from build123d import *

# Parameters (mm, degrees)
F0_R     = 10
F1_DEPTH = 30


with BuildPart() as f1:
    # F0 (on Front) → F1 (new body)
    with BuildSketch(Plane.XZ):
        Polygon((21.585897, 21.436766), (1.585897, 21.436766), (1.585897, 1.436766), (-16.747437, 1.436766), (-16.747437, -18.563234), (53.252563, -18.563234), (53.252563, -3.563234), (47.679901, 4.795761), (42.132899, 13.116264), (36.585897, 21.436766), (26.585897, 21.436766), (26.585897, 11.436766), (21.585897, 11.436766), align=None)
        with Locations((15.752563, -3.563234)):
            Circle(F0_R, mode=Mode.SUBTRACT)
        Polygon((49.066651, 29.757269), (36.585897, 21.436766), (42.132899, 13.116264), (54.613653, 21.436766), align=None)
        Polygon((47.679901, 4.795761), (53.252563, -3.563234), (65.733318, 4.757269), (60.160655, 13.116264), align=None)
    extrude(amount=F1_DEPTH)


solid = f1.part
Model file for the job. Use its own axes, mm. A direction names the side the tool comes from. Give positions to 0.01 mm unless a question says otherwise; leave off trailing zeros. Loops run counter-clockwise (first coordinate to the right, second up) from the corner with the lowest first, then second, coordinate; pieces in that order, holes last. Notation, with made-up numbers: (-38.75, 49.25) -> (13.25, 49.25) arc R14 cw to (13.25, 68.25) -> close; hole circle Ø1 at (-21, 86). An arc over 180 degrees is marked (long way). Use a Markdown table: item, result. Add a question column.
(1) Slice it at C-C on x = 24.5. List the corners of the cut face in (y, z).
(2) Tool access for faces 1 (the flat face through (21.586, -15, 16)), 2 (the flat face through (32, -15, 21.437)), 3 (the flat face through (54.008, -14.79, 9.014)): list every direction of +Z, -Z, +X, -X, +Y, -Y with a clear straight run to the whole face (end or side of a thin tool).
(3) Slice it at D-D on x = 0. List the corners of the cut face in (y, z).
(4) Drop flat-ended pins along their axis: pin 1 Ø10 at (y, z) = (-9.5, 12.5) entering from -X; pin 2 Ø8 at (x, y) = (29.5, -14) entering from +Z; pin 3 Ø1 at (y, z) = (-26.5, -13) entering from +X. Give the stop position or say it passes through.
(5) Mould opens along Z. For faces 4 (the flat face through (62.986, -14.79, 8.878)), 5 (the flat face through (24, -30, 6)), 6 (the flat face through (48.29, -14.79, 17.22)) say: +Z half, -Z half, draft (parallel to the pull), parting line (faces both ways), or undercut.
(6) Slice it at A-A on z = 16. List the corners of the cut face in (x, y).
(7) Wall check: line 1 along X through (y, z) = (-21.75, 12); line 2 along Z through (x, y) = (30.5, -21.75); line 3 along Z through (x, y) = (46, -23.5). Give the ranges that are in metal, low to high.
(8) Slice it at B-B on y = -22.75. List the corners of the cut face in (x, z), and give its area (3 significant figures).
Filled sheet:
| question | item | result |
|---|---|---|
| 1 | outline | (-30, -18.56) -> (0, -18.56) -> (0, -8.41) -> (-30, -8.41) -> close; (-30, 1.28) -> (0, 1.28) -> (0, 11.44) -> (-30, 11.44) -> close |
| 2 | face 1 | +Z, +Y, -Y |
| 2 | face 2 | +Z, -X, +Y, -Y |
| 2 | face 3 | +Y, -Y |
| 3 | outline | (-30, -18.56) -> (0, -18.56) -> (0, 1.44) -> (-30, 1.44) -> close |
| 4 | pin 1 | x = 1.59 |
| 4 | pin 2 | z = 21.44 |
| 4 | pin 3 | x = 53.25 |
| 5 | face 4 | +Z half |
| 5 | face 5 | draft |
| 5 | face 6 | undercut |
| 6 | outline | (1.59, -30) -> (21.59, -30) -> (21.59, 0) -> (1.59, 0) -> close; (26.59, -30) -> (46.46, -30) -> (46.46, 0) -> (26.59, 0) -> close |
| 7 | line 1 | 1.59 to 21.59, 26.59 to 42.88, 58.49 to 60.9 |
| 7 | line 2 | -18.56 to 21.44 |
| 7 | line 3 | -18.56 to 7.32, 15.69 to 27.71 |
| 8 | outline | (-16.75, -18.56) -> (53.25, -18.56) -> (53.25, -3.56) -> (65.73, 4.76) -> (60.16, 13.12) -> (47.68, 4.8) -> (42.13, 13.12) -> (54.61, 21.44) -> (49.07, 29.76) -> (36.59, 21.44) -> (26.59, 21.44) -> (26.59, 11.44) -> (21.59, 11.44) -> (21.59, 21.44) -> (1.59, 21.44) -> (1.59, 1.44) -> (-16.75, 1.44) -> close; hole circle Ø20 at (15.75, -3.56) |
| 8 | area | 2,160 mm2 |
